Build history of the part. All positions in model axes, mm. A direction names the side the tool comes from. Give positions to 0.01 mm unless a question says otherwise; leave off trailing zeros. Loops run counter-clockwise (first coordinate to the right, second up) from the corner with the lowest first, then second, coordinate; pieces in that order, holes last.
1) Band-saw the part on C-C on x = 217.5. List the corners of the cut face in (y, z) (3 decimals), then the cut area to 3 significant figures.
2) Band-saw the part on D-D on y = 204.5. List the corners of the cut face in (x, z).
3) Flat gauge pins, fed straight in: P1, Ø6, axis at x = 128.5, y = 199.5, coming from the +Z side; P2, Ø3, axis at y = 201.5, z = 142, coming from the -X side; P3, Ø10, axis at x = -30, y = 221, coming from the -Z side. Where does each tip first touch, or does it go through?
4) Band-saw the part on A-A on z = 0. List the corners of the cut face in (x, y) (3 decimals).
5) 3-axis set-ups, long thin cutter, end or side, ignore diameter. For faces 4 (the conical face through (-38.777, 137.821, -174.625)), 5 (the flat face through (4, 260.35, -174)): which of +Z, -Z, +X, -X, +Y, -Y reach the whole face in a straight line?
6) Band-saw the part on B-B on x = 0. List the corners of the cut face in (y, z) (3 decimals), then the cut area to 3 significant figures.
7) Two-plate mould, pull along Y, no slides. Class faces 1 (the cylindrical face through (254.384, 242.643, 80.109)), 2 (the flat face through (4, 0, -174)), 3 (the conical face through (-141.95, 122.53, -108.85)): +Y half, -Y half, draft (parallel to the pull), parting line (faces both ways), or undercut.
8) Wall check: line 1 (Z direction, x = 0, y = 132); line 2 (Y direction, x = 42.5, z = -208.5) (3 decimals); line 3 (X direction, y = 158.5, z = 110.5). Give the ranges that are in metal, low to high.
```python
from build123d import *

# Parameters (mm, degrees)
F4_W = 9.398
F4_H = 6.35


with BuildPart() as f1:
    # F0 (on Top) → F1 (revolve)
    with BuildSketch(Plane.XY):
        Polygon((168.402, 0), (266.7, 0), (266.7, 34.925), (200.025, 34.925), (177.8, 127), (168.402, 127), align=None)
    revolve(axis=Axis((0, 63.5, 0), (0, -1, 0)))



with BuildPart() as f3_1:
    # F3: instance of F1
    add(f1.part.mirror(Plane.XZ.offset(-130.175)))


with BuildPart() as f1_1:
    add(f1.part)

    add(f3_1.part)  # F5 merges F3_1
    # F4 (on Top) → F5 (revolve)
    with BuildSketch(Plane.XY):
        with Locations((173.101, 130.175)):
            Rectangle(F4_W, F4_H)
    revolve(axis=Axis((0, 63.5, 0), (0, -1, 0)))


solid = f1_1.part
```
Findings below:
1. outline: (0, -154.346) - (34.925, -154.346) - (34.925, 154.346) - (0, 154.346) - close; (225.425, -154.346) - (260.35, -154.346) - (260.35, 154.346) - (225.425, 154.346) - close
1. area: 21,600 mm2
2. outline: circle Ø389.95 at (0, 0); hole circle Ø336.8 at (0, 0)
3. P1: stops at z = 147.8
3. P2: stops at x = -134.22
3. P3: stops at z = -265.26
4. outline: (-266.7, 0) - (-168.402, 0) - (-168.402, 260.35) - (-266.7, 260.35) - (-266.7, 225.425) - (-200.025, 225.425) - (-177.8, 133.35) - (-177.8, 127) - (-200.025, 34.925) - (-266.7, 34.925) - close; (168.402, 0) - (266.7, 0) - (266.7, 34.925) - (200.025, 34.925) - (177.8, 127) - (177.8, 133.35) - (200.025, 225.425) - (266.7, 225.425) - (266.7, 260.35) - (168.402, 260.35) - close
5. face 4: none
5. face 5: +Z, -Z, +X, -X, +Y
6. outline: (0, -266.7) - (34.925, -266.7) - (34.925, -200.025) - (127, -177.8) - (133.35, -177.8) - (225.425, -200.025) - (225.425, -266.7) - (260.35, -266.7) - (260.35, -168.402) - (0, -168.402) - close; (0, 168.402) - (260.35, 168.402) - (260.35, 266.7) - (225.425, 266.7) - (225.425, 200.025) - (133.35, 177.8) - (127, 177.8) - (34.925, 200.025) - (34.925, 266.7) - (0, 266.7) - close
6. area: 21,400 mm2
7. face 1: draft
7. face 2: -Y half
7. face 3: undercut
8. line 1: z = -177.8 to -168.4, 168.4 to 177.8
8. line 2: y = 0 to 34.925, 225.425 to 260.35
8. line 3: x = -146.96 to -127.08, 127.08 to 146.96
